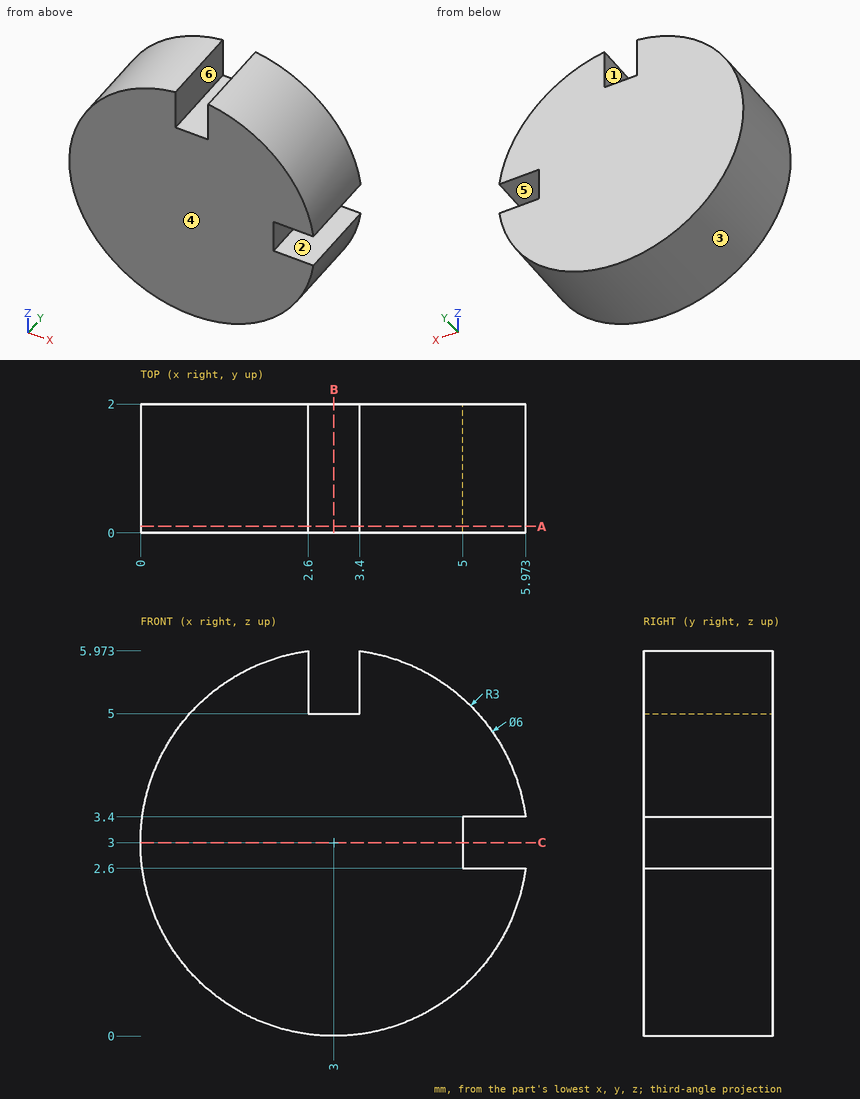
Here's the drawing with two shaded views (mm, measured from the low corner). I have some questions. A direction names the side the tool comes from. Give positions to 0.01 mm unless a question says otherwise; leave off trailing zeros. Order: outer loops, then holes, each group sorted by start corner. A loop starts at its lowest first (then second) coordinate and runs counter-clockwise, first axis right, second up.
Q1. I'm going to push flat-ended pins straight in: P1, Ø1.5, axis at x = 4, z = 1, coming from the -Y side; P2, Ø0.5, axis at x = 5.5, y = 1, coming from the -Z side (1 decimal); P3, Ø0.8, axis at y = 1, z = 5.5, coming from the -X side; P4, Ø0.8, axis at y = 1.5, z = 5.5, coming from the +X side. Where does each tip first touch, or does it pass through?
Q2. If I drill on line 1 along Z through (x, y) = (5.3, 1.6) (1 decimal); line 2 along X through (y, z) = (1.15, 5.45); line 3 along Z through (x, y) = (5.6, 0.3) (1 decimal), over which ranges is the centre line in solid material (lowest first)?
Q3. Suppose I cut it at A-A, the plane y = 0.1. Write out the boundary of the cut face in (x, z), and give its area (3 significant figures).
Q4. For the marked faces 4, 5 and 6, which set-ups out of +Z, -Z, +X, -X, +Y, -Y let a thin tool reach every point of the face, with its end or its side?
Q5. Suppose I cut it at B-B, the plane x = 3. Write out the boundary of the cut face in (y, z), and give its area (3 significant figures).
Q6. Suppose I cut it at C-C, the plane z = 3. Write out the boundary of the cut face in (x, y), and give its area (3 significant figures).
Q7. We'd pull the mould along X, two halves only. Please class the marked faces 1, 2 and 3: +X half, -X half, draft (parallel to the pull), parting line (faces both ways), or undercut.
Solution:
1. P1: stops at y = 0
1. P2: stops at z = 1
1. P3: stops at x = 0.86
1. P4: stops at x = 5.14
2. line 1: z = 1.1 to 2.6, 3.4 to 4.9
2. line 2: x = 1.27 to 2.6, 3.4 to 4.73
2. line 3: z = 1.5 to 2.6, 3.4 to 4.5
3. outline: (2.6, 5) - (2.6, 5.97) arc R3 ccw (long way) to (5.97, 2.6) - (5, 2.6) - (5, 3.4) - (5.97, 3.4) arc R3 ccw to (3.4, 5.97) - (3.4, 5) - close
3. area: 26.7 mm2
4. face 4: +Z, -Z, +X, -X, -Y
4. face 5: +X, +Y, -Y
4. face 6: +Z, +Y, -Y
5. outline: (0, 0) - (2, 0) - (2, 5) - (0, 5) - close
5. area: 10.0 mm2
6. outline: (0, 0) - (5, 0) - (5, 2) - (0, 2) - close
6. area: 10.0 mm2
7. face 1: undercut
7. face 2: draft
7. face 3: parting line
